Read the model definition and answer for the solid it produces. Units are mm, in the model's axes. A direction names the side the tool comes from. Give positions to 0.01 mm unless a question says otherwise; leave off trailing zeros. Order: outer loops, then holes, each group sorted by start corner. A loop starts at its lowest first (then second) coordinate and runs counter-clockwise, first axis right, second up. Notation, with made-up numbers: (-10.75, -39.75) - (19.25, -39.75) arc R9 cw to (19.25, -23.75) - close; hole circle Ø5 at (49.5, 26). An arc over 180 degrees is marked (long way). Answer as CSV lines item,"result". Start each with the question number.
from build123d import *

# Parameters (mm, degrees)
F0_W     = 434.975
F0_H     = 330.2
F1_DEPTH = 44.45
F2_R     = 3.4925
F3_DEPTH = 0.762
F5_DEPTH = 431.8
F6_W     = 395.026488
F6_H     = 25.4
F7_DEPTH = 88.901


with BuildPart() as f1:
    # F0 (on Top) → F1 (new body, symmetric)
    with BuildSketch(Plane.XY):
        Rectangle(F0_W, F0_H)
    extrude(amount=F1_DEPTH, both=True)

    # F2 (on face) → F3 (join)
    with BuildSketch(Plane.XZ.offset(165.1)):
        Polygon((-241.3, 44.45), (-241.3, -44.45), (-217.4875, -44.45), (241.3, -44.45), (241.3, 44.45), align=None)
        with Locations((-229.39375, -34.6075)):
            Circle(F2_R, mode=Mode.SUBTRACT)
        with Locations((229.39375, -34.6075)):
            Circle(F2_R, mode=Mode.SUBTRACT)
        with Locations((-229.39375, 34.6075)):
            Circle(F2_R, mode=Mode.SUBTRACT)
        with Locations((229.39375, 34.6075)):
            Circle(F2_R, mode=Mode.SUBTRACT)
    extrude(amount=F3_DEPTH)

    # F4 (on face) → F5 (join)
    with BuildSketch(Plane.YZ.offset(217.4875)):
        with BuildLine():
            Line((-191.262, 15.875), (-191.262, 0))
            Line((-191.262, 0), (-191.262, -15.875))
            ThreePointArc((-191.262, -15.875), (-187.542256, -24.855256), (-178.562, -28.575))
            Line((-178.562, -28.575), (-165.862, -28.575))
            Line((-165.862, -28.575), (-165.862, -26.035))
            Line((-165.862, -26.035), (-178.562, -26.035))
            ThreePointArc((-178.562, -26.035), (-185.746205, -23.059205), (-188.722, -15.875))
            Line((-188.722, -15.875), (-188.722, 0))
            Line((-188.722, 0), (-188.722, 15.875))
            ThreePointArc((-188.722, 15.875), (-185.746205, 23.059205), (-178.562, 26.035))
            Line((-178.562, 26.035), (-165.862, 26.035))
            Line((-165.862, 26.035), (-165.862, 28.575))
            Line((-165.862, 28.575), (-178.562, 28.575))
            ThreePointArc((-178.562, 28.575), (-187.542256, 24.855256), (-191.262, 15.875))
        make_face()
    extrude(amount=-F5_DEPTH)

    # F6 (on face) → F7 (cut, through all)
    with BuildSketch(Plane.XY.offset(44.45)):
        with Locations((4.099256, -178.562)):
            Rectangle(F6_W, F6_H)
    extrude(amount=-F7_DEPTH, mode=Mode.SUBTRACT)


solid = f1.part
(1) Section A-A, the plane z = -4.5 is taken. Write down the section's boundary in (x, y), and give its area (3 significant figures).
(2) Straight lines are drawn through the part: line 1 (Z direction, x = -194, y = -174) (3 decimals); line 2 (Y direction, x = 97.5, z = -13.5); line 3 (X direction, y = 123.5, z = -25). For each, find the intervals that lie inside material, in ascending order. Write a range as [from, to].
(3) Determine the mould class of faces 5 (the flat face through (-3, 2, -44.45)), 6 (the flat face through (201.612, -189, 0)), 7 (the flat face through (217.488, -2, 1)), 8 (the flat face through (-217.488, -2, 1)) for opening direction X: released by +X, released by -X, zero draft, split by the parting line, or undercut.
(4) Flat-ended cylindrical pins translate along their axes: pin 1 Ø1 at (y, z) = (-32, 29) entering from +X; pin 2 Ø12.5 at (y, z) = (-175.5, 1) entering from -X; pin 3 Ø1 at (x, z) = (-117, -7.5) entering from -Y; pin 4 Ø8 at (x, z) = (-229.39, -34.61) entering from +Y. Find the tip coordinate at first contact, or state that the pin passes through.
(5) Section C-C, the plane x = -36 is taken. Write down the section's boundary in (y, z).
(6) Section B-B, the plane y = 51 is taken. Write down the section's boundary in (x, z).
(7) Which of the six approach directions +Z, -Z, +X, -X, +Y, -Y give full straight-line access (tool end or side, diameter ignored) to faces 1 (the flat face through (-204, -172, 26.035)), 2 (the flat face through (-204, -172, 28.575)), 3 (the flat face through (-204, -172, -28.575)), 4 (the flat face through (210, -191.262, 0))?
Checks:
1,outline,"(-241.3, -165.86) - (241.3, -165.86) - (241.3, -165.1) - (217.49, -165.1) - (217.49, 165.1) - (-217.49, 165.1) - (-217.49, -165.1) - (-241.3, -165.1) - close; (-214.31, -191.26) - (-193.41, -191.26) - (-193.41, -188.72) - (-214.31, -188.72) - close; (201.61, -191.26) - (217.49, -191.26) - (217.49, -188.72) - (201.61, -188.72) - close"
1,area,"144,000 mm²"
2,line 1,"z = [-28.575, -26.035], [26.035, 28.575]"
2,line 2,"y = [-165.86, 165.1]"
2,line 3,"x = [-217.49, 217.49]"
3,face 5,"zero draft"
3,face 6,"undercut"
3,face 7,"released by +X"
3,face 8,"released by -X"
4,pin 1,"stops at x = 217.49"
4,pin 2,"passes through"
4,pin 3,"stops at y = -165.86"
4,pin 4,"stops at y = -165.1"
5,outline,"(-165.86, -44.45) - (165.1, -44.45) - (165.1, 44.45) - (-165.86, 44.45) - close"
6,outline,"(-217.49, -44.45) - (217.49, -44.45) - (217.49, 44.45) - (-217.49, 44.45) - close"
7,face 1,"+X, -X"
7,face 2,"+Z, +X, -X, -Y"
7,face 3,"-Z, +X, -X, -Y"
7,face 4,"+Z, -Z, +X, -X, -Y"
